```python
from build123d import *

# Parameters (mm, degrees)
BOSS_EXTRUDE1_DEPTH = 16
CHAMFER1_SIZE       = 10
CHAMFER1_SIZE2      = 7
SKETCH2_R           = 1.6
CUT_EXTRUDE1_DEPTH  = 35.267331381
CUT_EXTRUDE2_START  = -5
CUT_EXTRUDE2_DEPTH  = 30.267331381
FILLET1_R           = 1


with BuildPart() as part:
    # Sketch1 → Boss-Extrude1 (new body)
    with BuildSketch(Plane.XY):
        with BuildLine():
            Line((10.5, 0), (10.5, -10.5))
            Line((10.5, -10.5), (18.5, -10.5))
            Line((18.5, -10.5), (18.5, 13.5))
            Line((18.5, 13.5), (0, 13.5))
            ThreePointArc((0, 13.5), (-10.52842962, 8.449980458), (-13.180003635, -2.92190078))
            Line((-13.180003635, -2.92190078), (-11.5, -10.5))
            Line((-11.5, -10.5), (-11.5, -16.5))
            Line((-11.5, -16.5), (-12.697755895, -16.5))
            Line((-12.697755895, -16.5), (-12.697755895, -18.5))
            ThreePointArc((-12.697755895, -18.5), (-12.404862676, -19.207106781), (-11.697755895, -19.5))
            Line((-11.697755895, -19.5), (-8.5, -19.5))
            Line((-8.5, -19.5), (-8.5, -6.164414003))
            ThreePointArc((-8.5, -6.164414003), (-3.240370349, 9.987492178), (10.5, 0))
        make_face()
    extrude(amount=BOSS_EXTRUDE1_DEPTH)

    # Chamfer1
    chamfer1_edges = [part.edges().sort_by_distance(p)[0] for p in [
        (18.5, 13.5, 8),
    ]]
    chamfer1_side = [part.faces().sort_by_distance(p)[0] for p in [
        (18.5, 1.5, 8),
    ]]
    chamfer(chamfer1_edges, length=CHAMFER1_SIZE, length2=CHAMFER1_SIZE2, reference=chamfer1_side[0])

    # Sketch2 → Cut-Extrude1 (cut, through all)
    with BuildSketch(Plane.XZ.offset(10.5)):
        with Locations(Location((14.5, 8, 0), (0, 0, 270))):
            Circle(SKETCH2_R)
    extrude(amount=-CUT_EXTRUDE1_DEPTH, mode=Mode.SUBTRACT)

    # Sketch3 → Cut-Extrude2 (cut, through all)
    with BuildSketch(Plane.XZ.offset(10.5).offset(CUT_EXTRUDE2_START)):
        Polygon((17.25, 6.41228676), (19.609136336, 7.774334758), (19.609136336, 17.446849576), (11.75, 9.58771324), (11.75, 6.41228676), (14.5, 4.824573519), align=None)
    extrude(amount=-CUT_EXTRUDE2_DEPTH, mode=Mode.SUBTRACT)

    # Fillet1
    fillet1_edges = [part.edges().sort_by_distance(p)[0] for p in [
        (-8.5, -19.5, 8),
    ]]
    fillet(fillet1_edges, radius=FILLET1_R)


solid = part.part
```
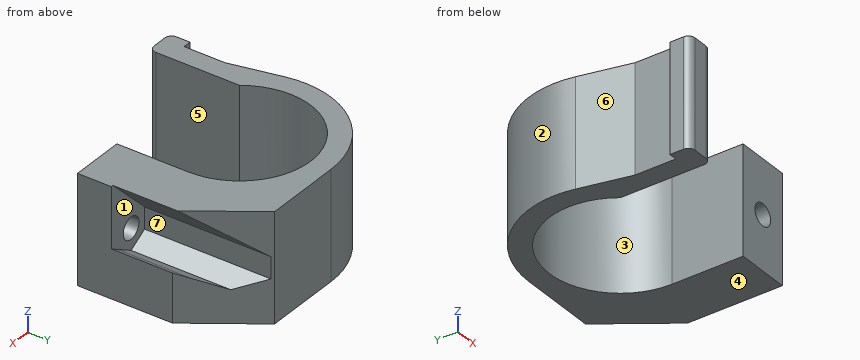
The listing builds one solid part. Answer for the finished solid, in the listing's coordinates (mm). Face numbers are marked on the shaded views. A direction names the side the tool comes from. Give positions to 0.01 mm unless a question says otherwise; leave off trailing zeros. Order: outer loops, then holes, each group sorted by start corner. A loop starts at its lowest first (then second) coordinate and runs counter-clockwise, first axis right, second up. Notation, with made-up numbers: (29.5, 50) -> (35.5, 50) arc R25 cw to (35.5, 88) -> close; hole circle Ø9 at (86, -7.75). An arc over 180 degrees is marked (long way). Answer as a JSON object with one key per item and string values. Group by question number.
Item 1: The part is cut by section D-D on x = 7. Write down the section's boundary in (y, z), and give its area (3 significant figures).
Item 2: The part is cut by section A-A on z = 8. Write down the section's boundary in (x, y), and give its area (3 significant figures).
Item 3: The part is cut by section C-C on z = 12.75. Write down the section's boundary in (x, y), and give its area (3 significant figures).
Item 4: The part is cut by section B-B on y = 10. Write down the section's boundary in (x, z), and give its area (3 significant figures).
Item 5: A tool of negligible diameter and unlimited length cuts with its end or side. For the marked faces 5, 6 and 7, from which of +Z, -Z, +X, -X, +Y, -Y can it reach the whole face along a straight path? Write none if from no direction.
Item 6: Determine the mould class of the marked faces 1, 2, 3 and 4 for opening direction X: pulls with the +X half, pulls with the -X half, needs draft (parallel to the pull), parting line crosses it, or undercut.
Item 7: Consider L1, parallel to X at y = -6.85, z = 8; L2, parallel to X at y = 4, z = 5; L3, parallel to X at y = 1, z = 11.5. Determine where each line is inside the solid, lowest interval first. Write a range as from..to.
Item 8: Flat-ended cylindrical pins translate along their axes: pin 1 (5.5 mm diameter, centred on x = 16, z = 11, fed in from +Y); pin 2 (2.5 mm diameter, centred on y = 1.5, z = 8.5, fed in from +X); pin 3 (1 mm diameter, centred on y = -17, z = 5, fed in from -X); pin 4 (6 mm diameter, centred on x = -2, z = 14, fed in from +Y). Find the tip coordinate at first contact, or state that the pin passes through.
Result set:
{
 "1": {"outline": "(7.83, 0) -> (13.5, 0) -> (13.5, 16) -> (7.83, 16) -> close", "area": "90.8 mm²"},
 "2": {"outline": "(-13.18, -2.92) -> (-11.5, -10.5) -> (-11.5, -16.5) -> (-12.7, -16.5) -> (-12.7, -18.5) arc R1 ccw to (-11.7, -19.5) -> (-9.5, -19.5) arc R1 ccw to (-8.5, -18.5) -> (-8.5, -6.16) arc R10.5 cw (long way) to (10.5, 0) -> (10.5, -10.5) -> (12.9, -10.5) -> (12.9, -5.5) -> (11.75, -5.5) -> (11.75, 13.14) -> (11.5, 13.5) -> (0, 13.5) arc R13.5 ccw to start; (16.1, -10.5) -> (18.5, -10.5) -> (18.5, -5.5) -> (16.1, -5.5) -> close", "area": "225 mm²"},
 "3": {"outline": "(-13.18, -2.92) -> (-11.5, -10.5) -> (-11.5, -16.5) -> (-12.7, -16.5) -> (-12.7, -18.5) arc R1 ccw to (-11.7, -19.5) -> (-9.5, -19.5) arc R1 ccw to (-8.5, -18.5) -> (-8.5, -6.16) arc R10.5 cw (long way) to (10.5, 0) -> (10.5, -10.5) -> (18.5, -10.5) -> (18.5, -5.5) -> (14.91, -5.5) -> (14.91, 8.63) -> (11.5, 13.5) -> (0, 13.5) arc R13.5 ccw to start", "area": "292 mm²"},
 "4": {"outline": "(-9.07, 0) -> (-3.2, 0) -> (-3.2, 16) -> (-9.07, 16) -> close; (3.2, 0) -> (13.95, 0) -> (13.95, 5.14) -> (11.75, 6.41) -> (11.75, 9.59) -> (13.95, 11.79) -> (13.95, 16) -> (3.2, 16) -> close", "area": "255 mm²"},
 "5": {"face 5": "+Z, -Z, -Y", "face 6": "+Z, -Z, -X", "face 7": "+Y"},
 "6": {"face 1": "undercut", "face 2": "pulls with the -X half", "face 3": "undercut", "face 4": "needs draft"},
 "7": {"L1": "-12.31..-8.5, 10.5..12.9, 16.1..18.5", "L2": "-12.89..-9.71, 9.71..14.2, 14.8..18.15", "L3": "-13.46..-10.45, 10.45..13.66"},
 "8": {"pin 1": "y = 11", "pin 2": "x = 11.91", "pin 3": "x = -12.7", "pin 4": "y = 13.5"}
}
